For this review, take the finished solid that the model builds, in its own axes (mm). A direction names the side the tool comes from. Give positions to 0.01 mm unless a question says otherwise; leave off trailing zeros. Order: outer loops, then holes, each group sorted by start corner. A loop starts at its lowest first (then second) coordinate and runs counter-clockwise, first axis right, second up. Notation, with made-up numbers: (43.5, 27) -> (57.5, 27) arc R20 ccw to (57.5, 36) -> close; hole circle Ø6 at (55, 10). An arc over 180 degrees is marked (long way). Return JSON: item names as keys, results as strings. Group by question number.
1) For faces 1 (the face through (1.325, -1.986, -1.277)), 2 (the face through (1.863, 1.331, -1.262)), 3 (the face through (-0.65, -0.49, 0.48)), list the 3-axis set-ups (+Z, -Z, +X, -X, +Y, -Y) from which the entire face can be reached by the end or side of a thin tool; tool diameter is ignored.
2) Insertion check: P1, Ø1.5, axis at x = -1, y = 1, coming from the +Z side; P2, Ø1.6, axis at x = -0.5, z = -0.5, coming from the +Y side; P3, Ø1, axis at y = 0.5, z = -2.5, coming from the +X side; P4, Ø3, axis at x = 1.5, y = -2, coming from the +Z side. Each pin has a flat end and moves straight along its axis. Give the tip position at first contact, or say it passes through.
3) Add section C-C (z = -0.65). Give the boundary of the cut face in (x, y).
4) Add section D-D (x = -1.35). Give the boundary of the cut face in (y, z).
5) To check wall thickness, follow line 1 along Y through (x, z) = (-1.2, -0.8); line 2 along X through (y, z) = (1.3, -1.85); line 3 along Y through (x, z) = (-2.7, -0.3). State the ranges of each line that lie inside material, in increasing order.
6) Add section B-B (x = -2.35). Give the boundary of the cut face in (y, z), then the cut area to 3 significant figures.
7) The part is to be moulded in two halves that separate along Y. For faces 4 (the face through (1.002, 1.961, 0.121)), 5 (the face through (0.3, -1, -1.4)), 6 (the face through (-1, 1.2, -1)), 7 (the face through (-1, -3, 0)), say which applies: released by +Y, released by -Y, zero draft, split by the parting line, or undercut.
8) Add section A-A (z = -1.75). Give the boundary of the cut face in (x, y), then the cut area to 3 significant figures.
from build123d import *

# Parameters (mm, degrees)
SKETCH1_R           = 2.5
BOSS_EXTRUDE1_DEPTH = 2.7
SKETCH1_3_R         = 2
BOSS_EXTRUDE2_DEPTH = 1
SKETCH5_R           = 1
BOSS_EXTRUDE3_DEPTH = 1
SKETCH6_R           = 2
BOSS_EXTRUDE4_DEPTH = 2
SKETCH12_R          = 1.65
CUT_EXTRUDE1_DEPTH  = 1.5


with BuildPart() as part:
    # Sketch1 → Boss-Extrude1 (new body)
    with BuildSketch(Plane(origin=(0, 0, 0), x_dir=(1, 0, 0), z_dir=(0, 1, 0))):
        with Locations((-0.522013312, 0.511138034)):
            Circle(SKETCH1_R)
    extrude(amount=BOSS_EXTRUDE1_DEPTH)

    # Sketch1<3> → Boss-Extrude2 (add)
    with BuildSketch(Plane(origin=(0, 0, 0), x_dir=(1, 0, 0), z_dir=(0, 1, 0))):
        with Locations((-0.522013312, 0.511138034)):
            Circle(SKETCH1_3_R)
    extrude(amount=BOSS_EXTRUDE2_DEPTH)

    # Sketch5 → Boss-Extrude3 (add)
    with BuildSketch(Plane.XZ):
        with Locations((-0.522013312, -0.511138034)):
            Circle(SKETCH5_R)
    extrude(amount=BOSS_EXTRUDE3_DEPTH)

    # Sketch6 → Boss-Extrude4 (add)
    with BuildSketch(Plane.XZ.offset(1)):
        with Locations((-0.522013312, -0.511138034)):
            Circle(SKETCH6_R)
    extrude(amount=BOSS_EXTRUDE4_DEPTH)

    # Sketch12 → Cut-Extrude1 (cut)
    with BuildSketch(Plane(origin=(0, 2.7, 0), x_dir=(1, 0, 0), z_dir=(0, 1, 0))):
        with Locations((-0.522013312, 0.511138034)):
            Circle(SKETCH12_R)
    extrude(amount=-CUT_EXTRUDE1_DEPTH, mode=Mode.SUBTRACT)


solid = part.part
Evaluation:
{
 "1": {"face 1": "-Y", "face 2": "+Y, -Y", "face 3": "none"},
 "2": {"P1": "z = 1.99", "P2": "y = 1.2", "P3": "x = 1.49", "P4": "z = 1.42"},
 "3": {"outline": "(-3.02, 0) -> (-1.51, 0) -> (-1.51, -1) -> (-2.52, -1) -> (-2.52, -3) -> (1.47, -3) -> (1.47, -1) -> (0.47, -1) -> (0.47, 0) -> (1.97, 0) -> (1.97, 2.7) -> (1.12, 2.7) -> (1.12, 1.2) -> (-2.17, 1.2) -> (-2.17, 2.7) -> (-3.02, 2.7) -> close"},
 "4": {"outline": "(-3, -2.33) -> (-1, -2.33) -> (-1, -1.07) -> (0, -1.07) -> (0, -2.87) -> (2.7, -2.87) -> (2.7, -1.94) -> (1.2, -1.94) -> (1.2, 0.92) -> (2.7, 0.92) -> (2.7, 1.85) -> (0, 1.85) -> (0, 0.05) -> (-1, 0.05) -> (-1, 1.31) -> (-3, 1.31) -> close"},
 "5": {"line 1": "-3 to 1.2", "line 2": "-2.63 to -1.49, 0.44 to 1.59", "line 3": "0 to 2.7"},
 "6": {"outline": "(-3, -1.32) -> (-1, -1.32) -> (-1, 0.3) -> (-3, 0.3) -> close; (0, -2.22) -> (2.7, -2.22) -> (2.7, 1.19) -> (0, 1.19) -> close", "area": "12.5 mm^2"},
 "7": {"face 4": "zero draft", "face 5": "undercut", "face 6": "released by +Y", "face 7": "released by -Y"},
 "8": {"outline": "(-2.69, 0) -> (1.65, 0) -> (1.65, 2.7) -> (0.57, 2.7) -> (0.57, 1.2) -> (-1.61, 1.2) -> (-1.61, 2.7) -> (-2.69, 2.7) -> close; (-2.09, -3) -> (1.05, -3) -> (1.05, -1) -> (-2.09, -1) -> close", "area": "14.7 mm^2"}
}
